from build123d import *

# Parameters (mm, degrees)
BOSS_EXTRUDE2_DEPTH   = 5
SKETCH3_R             = 4
BOSS_EXTRUDE3_DEPTH   = 22.5
SKETCH4_R             = 3
BOSS_EXTRUDE4_DEPTH   = 2
SKETCH5_R             = 4
BOSS_EXTRUDE5_DEPTH   = 2
F_6_CLEARANCE_HOLE1_D = 3.7973


with BuildPart() as part:
    # Sketch2 → Boss-Extrude2 (new body)
    with BuildSketch(Plane(origin=(0, 0, 0), x_dir=(1, 0, 0), z_dir=(0, 1, 0))):
        with BuildLine():
            ThreePointArc((-1.921673483, -7.798539123), (3.967844549, -11.837003018), (9.548776015, -7.381801872))
            Line((9.548776015, -7.381801872), (10.998470019, -1.926053578))
            ThreePointArc((10.998470019, -1.926053578), (11.24988985, -0.04064778), (11.018921171, 1.84737246))
            Line((11.018921171, 1.84737246), (9.565136937, 7.567628243))
            ThreePointArc((9.565136937, 7.567628243), (3.75, 12.089730275), (-2.065136937, 7.567628243))
            Line((-2.065136937, 7.567628243), (-3.518921171, 1.84737246))
            ThreePointArc((-3.518921171, 1.84737246), (-3.749830525, -0.050419155), (-3.493426606, -1.944934706))
            Line((-3.493426606, -1.944934706), (-1.921673483, -7.798539123))
        make_face()
    extrude(amount=BOSS_EXTRUDE2_DEPTH)

    # Sketch3 → Boss-Extrude3 (add)
    with BuildSketch(Plane(origin=(0, 5, 0), x_dir=(1, 0, 0), z_dir=(0, 1, 0))):
        with Locations(Location((3.75, -5.840959009, 0), (0, 0, 90))):
            Circle(SKETCH3_R)
        with Locations(Location((3.75, 6.089730275, 0), (0, 0, 90))):
            Circle(SKETCH3_R)
    extrude(amount=BOSS_EXTRUDE3_DEPTH)

    # Sketch4 → Boss-Extrude4 (add)
    with BuildSketch(Plane(origin=(0, 27.5, 0), x_dir=(1, 0, 0), z_dir=(0, 1, 0))):
        with Locations(Location((3.75, -5.840959009, 0), (0, 0, 270))):
            Circle(SKETCH4_R)
        with Locations(Location((3.75, 6.089730275, 0), (0, 0, 270))):
            Circle(SKETCH4_R)
    extrude(amount=BOSS_EXTRUDE4_DEPTH)

    # Sketch5 → Boss-Extrude5 (add)
    with BuildSketch(Plane(origin=(0, 29.5, 0), x_dir=(1, 0, 0), z_dir=(0, 1, 0))):
        with Locations(Location((3.75, -5.840959009, 0), (0, 0, 90))):
            Circle(SKETCH5_R)
        with Locations(Location((3.75, 6.089730275, 0), (0, 0, 90))):
            Circle(SKETCH5_R)
    extrude(amount=BOSS_EXTRUDE5_DEPTH)

    # #6 Clearance Hole1 (through all)
    with Locations(Plane(origin=(0, 5, 0), x_dir=(1, 0, 0), z_dir=(0, 1, 0))):
        with Locations((0, 0), (7.5, 0)):
            Hole(F_6_CLEARANCE_HOLE1_D / 2)


solid = part.part
The listing builds one solid part. Answer for the finished solid, in the listing's coordinates (mm). A direction names the side the tool comes from. Coordinates: 2 decimals unless noted, no trailing zeros. Write each loop counter-clockwise with the first axis right and the second up, starting at its lowest first coordinate (ties: lowest second). Pieces come first, ordered by that corner, then holes. Notation, with made-up numbers: (7, 24.5) - (62, 24.5) arc R18 cw to (62, 38.5) - close; hole circle Ø9 at (6.5, 23.5). An arc over 180 degrees is marked (long way). Return JSON: item names as keys, results as strings.
1. The part is cut by section A-A on z = 0. Determine the outline of the cut face in (x, y), then the cut area to 3 significant figures.
Final values:
{"outline": "(-3.75, 0) - (-1.9, 0) - (-1.9, 5) - (-3.75, 5) - close; (1.9, 0) - (5.6, 0) - (5.6, 5) - (1.9, 5) - close; (9.4, 0) - (11.25, 0) - (11.25, 5) - (9.4, 5) - close", "area": "37.0 mm^2"}
2. Which of the six approach directions +Z, -Z, +X, -X, +Y, -Y give full straight-line access (tool end or side, diameter ignored) to faces 4 (the face through (5.282, 30.486, -9.785)), 5 (the face through (10.263, 2.465, 4.692)), 6 (the face through (1, 27.5, 4))?
Final values:
{"face 4": "+Y", "face 5": "+Z, +X, +Y, -Y", "face 6": "none"}
3. The part is cut by section C-C on x = 3.75. Determine the outline of the cut face in (y, z).
Final values:
{"outline": "(0, -12.09) - (5, -12.09) - (5, -10.09) - (27.5, -10.09) - (27.5, -9.09) - (29.5, -9.09) - (29.5, -10.09) - (31.5, -10.09) - (31.5, -2.09) - (29.5, -2.09) - (29.5, -3.09) - (27.5, -3.09) - (27.5, -2.09) - (5, -2.09) - (5, 1.84) - (27.5, 1.84) - (27.5, 2.84) - (29.5, 2.84) - (29.5, 1.84) - (31.5, 1.84) - (31.5, 9.84) - (29.5, 9.84) - (29.5, 8.84) - (27.5, 8.84) - (27.5, 9.84) - (5, 9.84) - (5, 11.84) - (0, 11.84) - close"}
4. The part is cut by section D-D on z = -8.75. Determine the outline of the cut face in (x, y), then the cut area to 3 significant figures.
Final values:
{"outline": "(-1.63, 0) - (9.13, 0) - (9.13, 5) - (6.74, 5) - (6.74, 27.5) - (5.14, 27.5) - (5.14, 29.5) - (6.74, 29.5) - (6.74, 31.5) - (0.76, 31.5) - (0.76, 29.5) - (2.36, 29.5) - (2.36, 27.5) - (0.76, 27.5) - (0.76, 5) - (-1.63, 5) - close", "area": "206 mm^2"}
5. For a pull along Y with two mould halves and no side action, classify faces 1 (the face through (4, 31.5, -6)), 2 (the face through (1, 29.5, -8)), 3 (the face through (-2.72, 2.46, 4.83)) as +Y half, -Y half, draft (parallel to the pull), parting line (faces both ways), or undercut.
Final values:
{"face 1": "+Y half", "face 2": "undercut", "face 3": "draft"}
6. The part is cut by section B-B on y = 13.5. Determine the outline of the cut face in (x, z), then the cut area to 3 significant figures.
Final values:
{"outline": "circle Ø8 at (3.75, -6.09); circle Ø8 at (3.75, 5.84)", "area": "101 mm^2"}
7. Consider line 1 along Z through (x, y) = (3.5, 14); line 2 along Y through (x, z) = (4.25, -3); line 3 along X through (y, z) = (2, -0.5). Determine where each line is inside the solid, lowest interval first.
Final values:
{"line 1": "-10.08 to -2.1, 1.85 to 9.83", "line 2": "0 to 27.5, 29.5 to 31.5", "line 3": "-3.73 to -1.83, 1.83 to 5.67, 9.33 to 11.23"}
8. Each of these flat-tipped pins is pushed along its axis until it touches: pin 1 Ø1 at (x, y) = (-2, 15.5) entering from +Z; pin 2 Ø2 at (x, y) = (-0.5, 7) entering from -Z; pin 3 Ø8 at (x, y) = (9.5, 15) entering from +Z; pin 4 Ø5 at (x, y) = (3, 24.5) entering from -Z. Where does it stop, or does it pass through?
Final values:
{"pin 1": "through", "pin 2": "z = -8.42", "pin 3": "z = 9.44", "pin 4": "z = -10.09"}
